For this review, use the dimensioned drawing (mm, ordinates from the lowest corner) and the shaded views. A direction names the side the tool comes from. Coordinates: 2 decimals unless noted, no trailing zeros. Write each loop counter-clockwise with the first axis right and the second up, starting at its lowest first coordinate (ties: lowest second). Pieces come first, ordered by that corner, then holes.
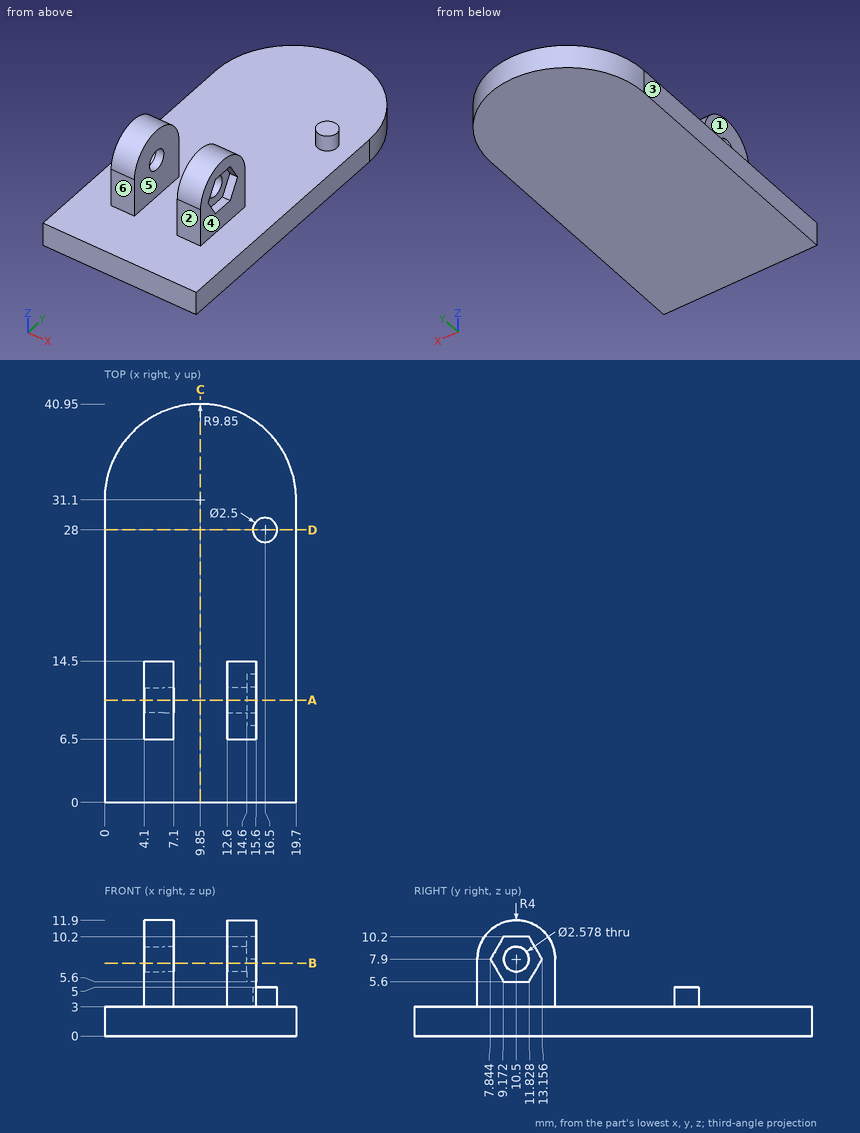
Item 1: Machinability: for the marked faces 1, 2 and 3, which of the approach directions +Z, -Z, +X, -X, +Y, -Y give a long, thin tool a straight path to every point of the face, cutting with its end or side? Answer none if there is none.
Solved:
face 1: +Z, -X, +Y, -Y
face 2: +Z, +X, -X, -Y
face 3: +Z, -Z, -X, +Y, -Y
Item 2: Mouldability with a two-part tool opening along X and no side actions: class the marked faces 4, 5 and 6 as pulls with the +X half, pulls with the -X half, needs draft (parallel to the pull), parting line crosses it, or undercut.
Solved:
face 4: pulls with the +X half
face 5: undercut
face 6: needs draft
Item 3: To check wall thickness, follow line 1 along Y through (x, z) = (6.7, 7.9); line 2 along Z through (x, y) = (14.1, 10.5); line 3 along X through (y, z) = (13.5, 10). State the ranges of each line that lie inside material, in increasing order.
Solved:
line 1: y = 6.5 to 9.21, 11.79 to 14.5
line 2: z = 0 to 6.61, 9.19 to 11.9
line 3: x = 4.1 to 7.1, 12.6 to 15.6
Item 4: Take a section at D-D, the plane y = 28. Write out the cut boundary in (x, z), plus the area to 3 significant figures.
Solved:
outline: (0, 0) - (19.7, 0) - (19.7, 3) - (17.75, 3) - (17.75, 5) - (15.25, 5) - (15.25, 3) - (0, 3) - close
area: 64.1 mm2
Item 5: Take a section at B-B, the plane z = 7.5. Write out the cut boundary in (x, y) (1 decimal).
Solved:
outline: (4.1, 6.5) - (7.1, 6.5) - (7.1, 9.3) - (4.1, 9.3) - close; (4.1, 11.7) - (7.1, 11.7) - (7.1, 14.5) - (4.1, 14.5) - close; (12.6, 6.5) - (15.6, 6.5) - (15.6, 8.1) - (14.6, 8.1) - (14.6, 9.3) - (12.6, 9.3) - close; (12.6, 11.7) - (14.6, 11.7) - (14.6, 12.9) - (15.6, 12.9) - (15.6, 14.5) - (12.6, 14.5) - close
Item 6: For pin 1 (6 mm diameter, centred on x = 13.5, y = 29, fed in from +Z); pin 2 (3 mm diameter, centred on x = 2.5, z = 9, fed in from +Y); pin 3 (6 mm diameter, centred on x = 8, y = 35.5, fed in from +Z); pin 4 (1.5 mm diameter, centred on x = 14, z = 5.5, fed in from -Y), all flat-tipped, find the tip position at first contact; note any pin that passes through.
Solved:
pin 1: stops at z = 5
pin 2: passes through
pin 3: stops at z = 3
pin 4: stops at y = 6.5
Item 7: Take a section at C-C, the plane x = 9.85. Write out the cut boundary in (y, z).
Solved:
outline: (0, 0) - (40.95, 0) - (40.95, 3) - (0, 3) - close
Item 8: Take a section at A-A, the plane y = 10.5. Write out the cut boundary in (x, z).
Solved:
outline: (0, 0) - (19.7, 0) - (19.7, 3) - (15.6, 3) - (15.6, 5.6) - (14.6, 5.6) - (14.6, 6.61) - (12.6, 6.61) - (12.6, 3) - (7.1, 3) - (7.1, 6.61) - (4.1, 6.61) - (4.1, 3) - (0, 3) - close; (4.1, 9.19) - (7.1, 9.19) - (7.1, 11.9) - (4.1, 11.9) - close; (12.6, 9.19) - (14.6, 9.19) - (14.6, 10.2) - (15.6, 10.2) - (15.6, 11.9) - (12.6, 11.9) - close
